Part print with two shaded views. Sizes in mm from the minimum x, y, z corner. A direction names the side the tool comes from. Coordinates: 2 decimals unless noted, no trailing zeros. Loops run counter-clockwise (first coordinate to the right, second up) from the corner with the lowest first, then second, coordinate; pieces in that order, holes last. Notation, with made-up numbers: (3, -28.75) -> (38, -28.75) arc R20 cw to (38, 10.25) -> close; hole circle Ø6 at (-26.5, 58.25). An arc over 180 degrees is marked (long way). Return JSON: item names as keys, results as strings. Group by question number.
(1) Flat gauge pins, fed straight in: pin 1 Ø2 at (x, y) = (5.5, 28.25) entering from -Z; pin 2 Ø0.8 at (x, z) = (2, 1) entering from -Y; pin 3 Ø0.8 at (y, z) = (28, 0.5) entering from +X. Where does each tip first touch, or does it go through?
(2) Saw through at D-D on x = 2.25. Write the cut outline in (y, z).
(3) Mould opens along X. For the marked faces 5, 6, 7 and 8 say: pulls with the +X half, pulls with the -X half, needs draft (parallel to the pull), parting line crosses it, or undercut.
(4) Probe L1, parallel to X at y = 1.75, z = 1; L2, parallel to Y at x = 5.5, z = 0.7; L3, parallel to Y at x = 1.75, z = 0.2. List the from-to ranges inside material, lowest first.
(5) Saw through at C-C on z = 0.7. Write the cut outline in (x, y).
(6) Saw through at A-A on x = 5.5. Write the cut outline in (y, z), then the cut area to 3 significant figures.
(7) Saw through at B-B on y = 28.25. Write the cut outline in (x, z).
(8) Tool access for the marked faces 1, 2, 3 and 4: list every direction of +Z, -Z, +X, -X, +Y, -Y with a clear straight run to the whole face (end or side of a thin tool).
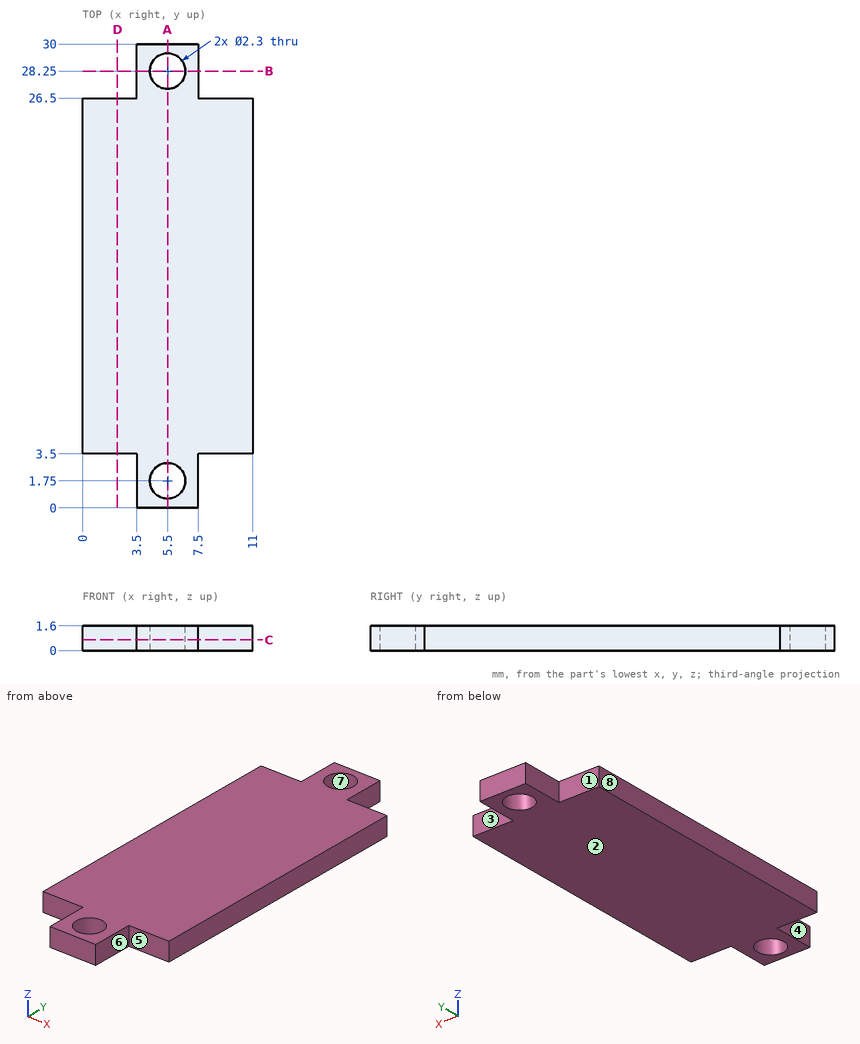
Geometry results:
{
 "1": {"pin 1": "through", "pin 2": "y = 3.5", "pin 3": "x = 7.5"},
 "2": {"outline": "(3.5, 0) -> (26.5, 0) -> (26.5, 1.6) -> (3.5, 1.6) -> close"},
 "3": {"face 5": "needs draft", "face 6": "pulls with the +X half", "face 7": "undercut", "face 8": "pulls with the -X half"},
 "4": {"L1": "3.5 to 4.35, 6.65 to 7.5", "L2": "0 to 0.6, 2.9 to 27.1, 29.4 to 30", "L3": "3.5 to 26.5"},
 "5": {"outline": "(0, 3.5) -> (3.5, 3.5) -> (3.5, 0) -> (7.5, 0) -> (7.5, 3.5) -> (11, 3.5) -> (11, 26.5) -> (7.5, 26.5) -> (7.5, 30) -> (3.5, 30) -> (3.5, 26.5) -> (0, 26.5) -> close; hole circle Ø2.3 at (5.5, 1.75); hole circle Ø2.3 at (5.5, 28.25)"},
 "6": {"outline": "(0, 0) -> (0.6, 0) -> (0.6, 1.6) -> (0, 1.6) -> close; (2.9, 0) -> (27.1, 0) -> (27.1, 1.6) -> (2.9, 1.6) -> close; (29.4, 0) -> (30, 0) -> (30, 1.6) -> (29.4, 1.6) -> close", "area": "40.6 mm²"},
 "7": {"outline": "(3.5, 0) -> (4.35, 0) -> (4.35, 1.6) -> (3.5, 1.6) -> close; (6.65, 0) -> (7.5, 0) -> (7.5, 1.6) -> (6.65, 1.6) -> close"},
 "8": {"face 1": "+Z, -Z, -X, +Y", "face 2": "-Z, +X, -X, +Y, -Y", "face 3": "+Z, -Z, +X, +Y", "face 4": "+Z, -Z, -X, -Y"}
}
